Design review of the part built by this model. Coordinates are the model's own, in mm. A direction names the side the tool comes from. Round coordinates to 2 decimals unless told otherwise and drop trailing zeros. Write each loop counter-clockwise with the first axis right and the second up, starting at its lowest first coordinate (ties: lowest second). Pieces come first, ordered by that corner, then holes. Notation, with made-up numbers: (58, 34) -> (107, 34) arc R19 ccw to (107, 65) -> close; hole circle Ø6 at (-25, 6.25). An arc over 180 degrees is marked (long way). One line per question, with ' | ' between items. Start each with the question number.
1) Mouldability with a two-part tool opening along Y and no side actions: class faces 1 (the flat face through (241, 29, 13)), 2 (the flat face through (248, 64.12, 8)), 3 (the cylindrical face through (32.235, 29.163, 27.04)) as +Y half, -Y half, draft (parallel to the pull), parting line (faces both ways), or undercut.
2) For faces 4 (the cylindrical face through (299.565, 57.612, 26.178)), 5 (the flat face through (253, 6, 0)), 6 (the flat face through (105, 57.52, 30)), 7 (the flat face through (253, 6, 60)), list the 3-axis set-ups (+Z, -Z, +X, -X, +Y, -Y) from which the entire face can be reached by the end or side of a thin tool; tool diameter is ignored.
3) Insertion check: pin 1 Ø2 at (x, z) = (314.82, 30.02) entering from +Y; pin 2 Ø6.5 at (y, z) = (54.5, 63.5) entering from -X; pin 3 Ø5 at (y, z) = (53.5, 30.5) entering from -X; pin 4 Ø1 at (x, y) = (68, 13.5) entering from -Z. Each pin has a flat end and moves straight along its axis. Give the tip position at first contact, or say it passes through.
4) Consider section A-A (y = 35). Count the separate pieces of the cut face and the enclosed holes in it, then the cut area to 3 significant figures.
5) For probe 1 along X at (y, z) = (52, -2.5); probe 2 along X at (y, z) = (55, 32); probe 3 along Y at (x, z) = (239.5, -5), list the stretches that pass through material, from the lowest coordinate up.
6) Consider section B-B (x = 186). Give the boundary of the cut face in (y, z).
```python
from build123d import *

# Parameters (mm, degrees)
SKETCH_1_W           = 300
SKETCH_1_H           = 60
EXTRUDE_1_DEPTH      = 57.52
FILLET_1_RADIUS      = 30
FILLET_1_LENGTH      = 57.52
SKETCH_9_W           = 60
SKETCH_9_H           = 44.32
CUT_EXTRUDE_5_DEPTH  = 59
FILLET_2_RADIUS      = 30
FILLET_2_LENGTH      = 6.6
FILLET_3_RADIUS      = 30
FILLET_3_LENGTH      = 6.6
SKETCH_10_R          = 29.5
CUT_EXTRUDE_6_DEPTH  = 51
FILLET_4_R           = 10
SKETCH_16_R          = 1.75
CUT_EXTRUDE_8_DEPTH  = 115
SKETCH_17_W          = 96.5
SKETCH_17_H          = 96.5
EXTRUDE_3_DEPTH      = 6.6
SKETCH_18_R          = 4
CUT_EXTRUDE_9_DEPTH  = 113.6
CUT_EXTRUDE_START    = -109
SKETCH_20_R          = 1.75
CUT_EXTRUDE_10_DEPTH = 109
SKETCH_21_R          = 29.5
CUT_EXTRUDE_11_DEPTH = 27
EXTRUDE_START        = -10
SKETCH_24_W          = 96.5
SKETCH_24_H          = 96.5
SKETCH_24_R          = 29.5
EXTRUDE_5_DEPTH      = 10
SKETCH_25_R          = 1.75
CUT_EXTRUDE_12_DEPTH = 28
SKETCH_26_R          = 4
CUT_EXTRUDE_13_DEPTH = 81
SKETCH_27_R          = 2
CUT_EXTRUDE_14_DEPTH = 57.52
SKETCH_28_R          = 4
CUT_EXTRUDE_15_DEPTH = 6.52
FILLET_5_R           = 10
FILLET_6_R           = 10
FILLET_7_R           = 10
FILLET_8_R           = 10
FILLET_10_R          = 10


with BuildPart() as part:
    # 草图1 → 凸台-拉伸1 (new body)
    with BuildSketch(Plane(origin=(0, 0, 0), x_dir=(1, 0, 0), z_dir=(0, 1, 0))):
        with Locations((150, -30)):
            Rectangle(SKETCH_1_W, SKETCH_1_H)
    extrude(amount=EXTRUDE_1_DEPTH)

    # 圆角1: full round fillet: the end face becomes a half cylinder, R = half its width
    fillet_1_face = Plane((0, 28.76, 30), x_dir=(0, -1, 0), z_dir=(-1, 0, 0))  # on the end face: x along it, z out of the body
    fillet_1_slab = fillet_1_face.offset(-FILLET_1_RADIUS / 2) * Box(FILLET_1_LENGTH, 2 * FILLET_1_RADIUS, FILLET_1_RADIUS, mode=Mode.PRIVATE)  # the body's end, R deep
    fillet_1_round = Plane((30, 28.76, 30), x_dir=(-1, 0, 0), z_dir=(0, -1, 0)) * Cylinder(FILLET_1_RADIUS, FILLET_1_LENGTH, mode=Mode.PRIVATE)  # its axis R under the face
    add(fillet_1_slab - fillet_1_round, mode=Mode.SUBTRACT)

    # 草图9 → 切除-拉伸5 (cut)
    with BuildSketch(Plane(origin=(300, 0, 0), x_dir=(0, 0, -1), z_dir=(1, 0, 0))):
        with Locations((-30, 28.76)):
            Rectangle(SKETCH_9_W, SKETCH_9_H)
    extrude(amount=-CUT_EXTRUDE_5_DEPTH, mode=Mode.SUBTRACT)

    # 圆角2: full round fillet: the end face becomes a half cylinder, R = half its width
    fillet_2_face = Plane((300, 54.22, 30), x_dir=(0, 1, 0), z_dir=(1, 0, 0))  # on the end face: x along it, z out of the body
    fillet_2_slab = fillet_2_face.offset(-FILLET_2_RADIUS / 2) * Box(FILLET_2_LENGTH, 2 * FILLET_2_RADIUS, FILLET_2_RADIUS, mode=Mode.PRIVATE)  # the body's end, R deep
    fillet_2_round = Plane((270, 54.22, 30), x_dir=(1, 0, 0), z_dir=(0, 1, 0)) * Cylinder(FILLET_2_RADIUS, FILLET_2_LENGTH, mode=Mode.PRIVATE)  # its axis R under the face
    add(fillet_2_slab - fillet_2_round, mode=Mode.SUBTRACT)

    # 圆角3: full round fillet: the end face becomes a half cylinder, R = half its width
    fillet_3_face = Plane((300, 3.3, 30), x_dir=(0, 1, 0), z_dir=(1, 0, 0))  # on the end face: x along it, z out of the body
    fillet_3_slab = fillet_3_face.offset(-FILLET_3_RADIUS / 2) * Box(FILLET_3_LENGTH, 2 * FILLET_3_RADIUS, FILLET_3_RADIUS, mode=Mode.PRIVATE)  # the body's end, R deep
    fillet_3_round = Plane((270, 3.3, 30), x_dir=(1, 0, 0), z_dir=(0, 1, 0)) * Cylinder(FILLET_3_RADIUS, FILLET_3_LENGTH, mode=Mode.PRIVATE)  # its axis R under the face
    add(fillet_3_slab - fillet_3_round, mode=Mode.SUBTRACT)

    # 草图10 → 切除-拉伸6 (cut)
    with BuildSketch(Plane(origin=(0, 57.52, 0), x_dir=(1, 0, 0), z_dir=(0, 1, 0))):
        with Locations(Location((270.132203493, -30.03743589, 0), (0, 0, 270))):
            Circle(SKETCH_10_R)
    extrude(amount=-CUT_EXTRUDE_6_DEPTH, mode=Mode.SUBTRACT)

    # 圆角4
    fillet_4_edges = [part.edges().sort_by_distance(p)[0] for p in [
        (241, 28.76, 34.681218791),
        (241, 28.76, 25.39365299),
    ]]
    fillet(fillet_4_edges, radius=FILLET_4_R)

    # 草图16 → 切除-拉伸8 (cut)
    with BuildSketch(Plane(origin=(0, 6.52, 0), x_dir=(1, 0, 0), z_dir=(0, 1, 0))):
        with Locations(Location((225.816101747, -30.018717945, 0), (0, 0, 90))):
            Circle(SKETCH_16_R)
    extrude(amount=CUT_EXTRUDE_8_DEPTH, mode=Mode.SUBTRACT)

    # 草图17 → 凸台-拉伸3 (add)
    with BuildSketch(Plane(origin=(0, 57.52, 0), x_dir=(1, 0, 0), z_dir=(0, 1, 0))):
        with Locations((270.316101747, -30.018717945)):
            Rectangle(SKETCH_17_W, SKETCH_17_H)
    extrude(amount=EXTRUDE_3_DEPTH)

    # 草图18 → 切除-拉伸9 (cut)
    with BuildSketch(Plane(origin=(0, 64.12, 0), x_dir=(1, 0, 0), z_dir=(0, 1, 0))):
        with Locations(Location((270.316101747, -12.768717945, 0), (0, 0, 270))):
            Circle(SKETCH_18_R)
        with Locations(Location((285.255039962, -21.393717945, 0), (0, 0, 270))):
            Circle(SKETCH_18_R)
        with Locations(Location((285.255039962, -38.643717945, 0), (0, 0, 270))):
            Circle(SKETCH_18_R)
        with Locations(Location((270.316101747, -47.268717945, 0), (0, 0, 270))):
            Circle(SKETCH_18_R)
        with Locations(Location((255.377163531, -38.643717945, 0), (0, 0, 270))):
            Circle(SKETCH_18_R)
        with Locations(Location((255.377163531, -21.393717945, 0), (0, 0, 270))):
            Circle(SKETCH_18_R)
    extrude(amount=-CUT_EXTRUDE_9_DEPTH, mode=Mode.SUBTRACT)

    # 草图20 → 切除-拉伸10 (cut)
    with BuildSketch(Plane(origin=(0, 64.12, 0), x_dir=(1, 0, 0), z_dir=(0, 1, 0)).offset(CUT_EXTRUDE_START)):
        with Locations(Location((270.316101747, 14.481282055, 0), (0, 0, 270))):
            Circle(SKETCH_20_R)
        with Locations(Location((301.782353509, 1.447533818, 0), (0, 0, 270))):
            Circle(SKETCH_20_R)
        with Locations(Location((314.816101747, -30.018717945, 0), (0, 0, 270))):
            Circle(SKETCH_20_R)
        with Locations(Location((301.782353509, -61.484969708, 0), (0, 0, 270))):
            Circle(SKETCH_20_R)
        with Locations(Location((270.316101747, -74.518717945, 0), (0, 0, 270))):
            Circle(SKETCH_20_R)
        with Locations(Location((238.849849984, -61.484969708, 0), (0, 0, 270))):
            Circle(SKETCH_20_R)
        with Locations(Location((225.816101747, -30.018717945, 0), (0, 0, 90))):
            Circle(SKETCH_20_R)
        with Locations(Location((238.849849984, 1.447533818, 0), (0, 0, 270))):
            Circle(SKETCH_20_R)
    extrude(amount=CUT_EXTRUDE_10_DEPTH, mode=Mode.SUBTRACT)

    # 草图21 → 切除-拉伸11 (cut)
    with BuildSketch(Plane(origin=(0, 64.12, 0), x_dir=(1, 0, 0), z_dir=(0, 1, 0))):
        with Locations(Location((270.316101747, -30.018717945, 0), (0, 0, 270))):
            Circle(SKETCH_21_R)
    extrude(amount=-CUT_EXTRUDE_11_DEPTH, mode=Mode.SUBTRACT)

    # 草图24 → 凸台-拉伸5 (add)
    with BuildSketch(Plane(origin=(0, 50.92, 0), x_dir=(-1, 0, 0), z_dir=(0, -1, 0)).offset(EXTRUDE_START)):
        with Locations((-270.316101747, -30.018717945)):
            Rectangle(SKETCH_24_W, SKETCH_24_H)
        with Locations(Location((-270.316101747, -30.018717945, 0), (0, 0, 270))):
            Circle(SKETCH_24_R, mode=Mode.SUBTRACT)
    extrude(amount=EXTRUDE_5_DEPTH)

    # 草图25 → 切除-拉伸12 (cut)
    with BuildSketch(Plane(origin=(0, 50.92, 0), x_dir=(-1, 0, 0), z_dir=(0, -1, 0))):
        with Locations(Location((-314.816101747, -30.018717945, 0), (0, 0, 270))):
            Circle(SKETCH_25_R)
        with Locations(Location((-301.782353509, 1.447533818, 0), (0, 0, 270))):
            Circle(SKETCH_25_R)
        with Locations(Location((-270.316101747, 14.481282055, 0), (0, 0, 270))):
            Circle(SKETCH_25_R)
        with Locations(Location((-238.849849984, 1.447533818, 0), (0, 0, 270))):
            Circle(SKETCH_25_R)
        with Locations(Location((-225.816101747, -30.018717945, 0), (0, 0, 90))):
            Circle(SKETCH_25_R)
        with Locations(Location((-238.849849984, -61.484969708, 0), (0, 0, 270))):
            Circle(SKETCH_25_R)
        with Locations(Location((-270.316101747, -74.518717945, 0), (0, 0, 270))):
            Circle(SKETCH_25_R)
        with Locations(Location((-301.782353509, -61.484969708, 0), (0, 0, 270))):
            Circle(SKETCH_25_R)
    extrude(amount=-CUT_EXTRUDE_12_DEPTH, mode=Mode.SUBTRACT)

    # 草图26 → 切除-拉伸13 (cut)
    with BuildSketch(Plane(origin=(0, 57.52, 0), x_dir=(1, 0, 0), z_dir=(0, 1, 0))):
        with Locations(Location((29.531429568, -29.988572589, 0), (0, 0, 270))):
            Circle(SKETCH_26_R)
    extrude(amount=-CUT_EXTRUDE_13_DEPTH, mode=Mode.SUBTRACT)

    # 草图27 → 切除-拉伸14 (cut)
    with BuildSketch(Plane(origin=(0, 57.52, 0), x_dir=(1, 0, 0), z_dir=(0, 1, 0))):
        with Locations(Location((29.531429568, -12.738572589, 0), (0, 0, 270))):
            Circle(SKETCH_27_R)
        with Locations(Location((44.470367783, -21.363572589, 0), (0, 0, 270))):
            Circle(SKETCH_27_R)
        with Locations(Location((44.470367783, -38.613572589, 0), (0, 0, 270))):
            Circle(SKETCH_27_R)
        with Locations(Location((29.531429568, -47.238572589, 0), (0, 0, 270))):
            Circle(SKETCH_27_R)
        with Locations(Location((14.592491352, -38.613572589, 0), (0, 0, 270))):
            Circle(SKETCH_27_R)
        with Locations(Location((14.592491352, -21.363572589, 0), (0, 0, 270))):
            Circle(SKETCH_27_R)
    extrude(amount=-CUT_EXTRUDE_14_DEPTH, mode=Mode.SUBTRACT)

    # 草图28 → 切除-拉伸15 (cut)
    with BuildSketch(Plane(origin=(0, 0, 0), x_dir=(-1, 0, 0), z_dir=(0, -1, 0))):
        with Locations(Location((-270.316101747, -30.018717945, 0), (0, 0, 90))):
            Circle(SKETCH_28_R)
    extrude(amount=-CUT_EXTRUDE_15_DEPTH, mode=Mode.SUBTRACT)

    # 圆角5
    fillet_5_edges = [part.edges().sort_by_distance(p)[0] for p in [
        (222.066101747, 57.52, -18.231282055),
    ]]
    fillet(fillet_5_edges, radius=FILLET_5_R)

    # 圆角6
    fillet_6_edges = [part.edges().sort_by_distance(p)[0] for p in [
        (318.566101747, 57.52, -18.231282055),
    ]]
    fillet(fillet_6_edges, radius=FILLET_6_R)

    # 圆角7
    fillet_7_edges = [part.edges().sort_by_distance(p)[0] for p in [
        (318.566101747, 57.52, 78.268717945),
    ]]
    fillet(fillet_7_edges, radius=FILLET_7_R)

    # 圆角8
    fillet_8_edges = [part.edges().sort_by_distance(p)[0] for p in [
        (222.066101747, 57.52, 78.268717945),
    ]]
    fillet(fillet_8_edges, radius=FILLET_8_R)

    # 圆角10
    # the kernel refuses this fillet: 10 mm, written as the material it adds along each edge
    with BuildSketch(Plane(origin=(222.066101747, 57.52, 60), x_dir=(0, 1, 0), z_dir=(0, 0, -1))) as fillet_10_piece_1:
        with BuildLine():
            CenterArc((10, -9.404254356), FILLET_10_R, 109.87687407, 70.12312593)
            Line((0, -9.404254356), (-0.2, -9.404254356))
            Line((-0.2, -9.404254356), (-0.2, 0))
            Line((-0.2, 0), (0, 0.2))
            ThreePointArc((0, 0.2), (3.3, 0.2), (6.532, 0.188085087))
            Line((6.532, 0.188085087), (6.6, 0))
        make_face()
    extrude(amount=60)


solid = part.part
```
From the geometry:
1) face 1: undercut | face 2: +Y half | face 3: draft
2) face 4: +Y | face 5: -Z, +X, -X, -Y | face 6: +Z, -Z, -X, +Y | face 7: +Z, +X, -X, -Y
3) pin 1: passes through | pin 2: stops at x = 222.07 | pin 3: stops at x = 0 | pin 4: stops at z = 0
4) separate pieces: 1 | enclosed holes: 8 | area: 13,900 mm2
5) probe 1: x = 222.07 to 237.45, 240.25 to 300.38, 303.18 to 318.57 | probe 2: x = 0.07 to 26.07, 32.99 to 240.88, 299.75 to 318.57 | probe 3: y = 50.92 to 64.12
6) outline: (0, 0) -> (57.52, 0) -> (57.52, 60) -> (0, 60) -> close
